```python
from build123d import *

# Parameters (mm, degrees)
F0_R     = 5
F0_W     = 10
F0_H     = 30
F1_DEPTH = 10
F2_DEPTH = 35
F3_R     = 14.99999
F5_D     = 10


# Not quite as in the source:
# - a fillet or chamfer is up to 0.001 mm smaller than in the source, because OpenCascade refuses the exact size


with BuildPart() as f1:
    # F0 (on Top) → F1 (new body)
    with BuildSketch(Plane.XY):
        with BuildLine():
            ThreePointArc((-20, 15), (-35, 0), (-20, -15))
            Line((-20, -15), (-5, -15))
            Line((-5, -15), (-5, 15))
            Line((-5, 15), (-20, 15))
        make_face()
        with Locations((-20, 0)):
            Circle(F0_R, mode=Mode.SUBTRACT)
        with BuildLine():
            Line((5, 15), (5, -15))
            Line((5, -15), (20, -15))
            ThreePointArc((20, -15), (35, 0), (20, 15))
            Line((20, 15), (5, 15))
        make_face()
        with Locations((20, 0)):
            Circle(F0_R, mode=Mode.SUBTRACT)
        Rectangle(F0_W, F0_H)
    extrude(amount=F1_DEPTH)

    # F0 (on Top) → F2 (join)
    with BuildSketch(Plane.XY):
        Rectangle(F0_W, F0_H)
    extrude(amount=F2_DEPTH)

    # F3 (radius 15 in the source; OpenCascade refuses exactly that, so slightly less here)
    f3_edges = [f1.edges().sort_by_distance(p)[0] for p in [
        (0, -15, 35),
        (0, 15, 35),
    ]]
    fillet(f3_edges, radius=F3_R)

    # F5 (through all)
    with Locations(Plane.YZ.offset(5)):
        with Locations((0, 20)):
            Hole(F5_D / 2)


solid = f1.part
```
Source: CAD feature listing. Evaluate the final solid. Frame: model axes, mm. A direction names the side the tool comes from. Round coordinates to 2 decimals unless told otherwise and drop trailing zeros. Loops run counter-clockwise (first coordinate to the right, second up) from the corner with the lowest first, then second, coordinate; pieces in that order, holes last.
1. Section query B-B on y = 2.5. Output: boundary loops of the cut face in (x, z), and give its area (3 significant figures).
2. Ray query, L1, parallel to Y at x = 20, z = 2.25; L2, parallel to Z at x = 0, y = 0; L3, parallel to X at y = 3, z = 5. Return the intervals inside material, ascending.
3. Contact query for flat-ended pins moving along their axis: pin 1 (12.5 mm diameter, centred on y = 2.5, z = 25, fed in from +X); pin 2 (9 mm diameter, centred on x = 25, y = 3.5, fed in from +Z); pin 3 (1.5 mm diameter, centred on y = 7, z = 7.5, fed in from +X). Output: stop coordinate, or through.
4. Section query D-D on z = 9. Output: boundary loops of the cut face in (x, y).
5. Mould query, pull axis Z, two halves, no side actions, for faces 3 (the flat face through (-5, 3, 25)), 4 (the cylindrical face through (-0.07, 1.08, 15.12)), 5 (the flat face through (-14, 0, 10)). Classes: released by +Z, released by -Z, zero draft, split by the parting line, or undercut.
6. Section query A-A on z = 21.5. Output: boundary loops of the cut face in (x, y), and give its area (3 significant figures).
7. Section query C-C on y = 12. Output: boundary loops of the cut face in (x, z), and give its area (3 significant figures).
8. Access query for faces 1 (the flat face through (16, 4, 10)), 2 (the cylindrical face through (-25, 0, 5)). Directions: +Z, -Z, +X, -X, +Y, -Y. A direction counts if a zero-diameter tool reaches every point of the face in a straight line with its end or side. Return the directions, or none.
Answers below:
1. outline: (-34.79, 0) - (-24.33, 0) - (-24.33, 10) - (-34.79, 10) - close; (-15.67, 0) - (15.67, 0) - (15.67, 10) - (5, 10) - (5, 15.67) - (-5, 15.67) - (-5, 10) - (-15.67, 10) - close; (-5, 24.33) - (5, 24.33) - (5, 34.79) - (-5, 34.79) - close; (24.33, 0) - (34.79, 0) - (34.79, 10) - (24.33, 10) - close
1. area: 684 mm2
2. L1: y = -15 to -5, 5 to 15
2. L2: z = 0 to 15, 25 to 35
2. L3: x = -34.7 to -24, -16 to 16, 24 to 34.7
3. pin 1: stops at x = 5
3. pin 2: stops at z = 10
3. pin 3: stops at x = 33.64
4. outline: (-20, -15) - (20, -15) arc R15 ccw to (20, 15) - (-20, 15) arc R15 ccw to start; hole circle Ø10 at (-20, 0); hole circle Ø10 at (20, 0)
5. face 3: zero draft
5. face 4: undercut
5. face 5: released by +Z
6. outline: (-5, -14.92) - (5, -14.92) - (5, -4.77) - (-5, -4.77) - close; (-5, 4.77) - (5, 4.77) - (5, 14.92) - (-5, 14.92) - close
6. area: 203 mm2
7. outline: (-29, 0) - (29, 0) - (29, 10) - (5, 10) - (5, 29) - (-5, 29) - (-5, 10) - (-29, 10) - close
7. area: 770 mm2
8. face 1: +Z, +X, +Y, -Y
8. face 2: +Z, -Z
